Geometry: final body of the model. Coordinates: model frame, mm. A direction names the side the tool comes from. Give positions to 0.01 mm unless a question says otherwise; leave off trailing zeros. Order: outer loops, then holes, each group sorted by start corner. A loop starts at its lowest first (then second) coordinate and runs counter-clockwise, first axis right, second up. Notation, with made-up numbers: (69, 26) -> (81, 26) arc R9 ccw to (81, 36) -> close; hole circle Ø8 at (59, -36). An arc over 180 degrees is marked (long way). One line per question, with ' | ' between items.
from build123d import *

# Parameters (mm, degrees)
SKETCH_1_R          = 31.5
EXTRUDE_1_DEPTH     = 25
SKETCH_2_R          = 5
EXTRUDE_2_DEPTH     = 9
SKETCH_3_R          = 31.5
EXTRUDE_3_DEPTH     = 4
SKETCH_4_R          = 29.5
CUT_EXTRUDE_1_DEPTH = 2
SKETCH_5_R          = 8
EXTRUDE_4_DEPTH     = 30
SKETCH_6_R          = 2
CUT_EXTRUDE_2_DEPTH = 20


with BuildPart() as part:
    # 草图1 → 凸台-拉伸1 (new body)
    with BuildSketch(Plane.XY):
        Circle(SKETCH_1_R)
    extrude(amount=EXTRUDE_1_DEPTH)

    # 草图2 → 凸台-拉伸2 (add)
    with BuildSketch(Plane.XY.offset(25)):
        Circle(SKETCH_2_R)
    extrude(amount=EXTRUDE_2_DEPTH)

    # 草图3 → 凸台-拉伸3 (add)
    with BuildSketch(Plane.XY.offset(34)):
        Circle(SKETCH_3_R)
    extrude(amount=EXTRUDE_3_DEPTH)

    # 草图4 → 切除-拉伸1 (cut)
    with BuildSketch(Plane.XY.offset(38)):
        Circle(SKETCH_4_R)
    extrude(amount=-CUT_EXTRUDE_1_DEPTH, mode=Mode.SUBTRACT)

    # 草图5 → 凸台-拉伸4 (add)
    with BuildSketch(Plane.XY.offset(36)):
        Circle(SKETCH_5_R)
    extrude(amount=EXTRUDE_4_DEPTH)

    # 草图6 → 切除-拉伸2 (cut, symmetric)
    with BuildSketch(Plane(origin=(0, 0, 0), x_dir=(1, 0, 0), z_dir=(0, 1, 0))):
        with Locations(Location((0, -58, 0), (0, 0, 270))):
            Circle(SKETCH_6_R)
    extrude(amount=CUT_EXTRUDE_2_DEPTH, both=True, mode=Mode.SUBTRACT)


solid = part.part
1) Section B-B on x = 0. Return loops of the section in (y, z), plus the area to 4 significant figures.
Check result:
outline: (-31.5, 0) -> (31.5, 0) -> (31.5, 25) -> (5, 25) -> (5, 34) -> (31.5, 34) -> (31.5, 38) -> (29.5, 38) -> (29.5, 36) -> (8, 36) -> (8, 56) -> (-8, 56) -> (-8, 36) -> (-29.5, 36) -> (-29.5, 38) -> (-31.5, 38) -> (-31.5, 34) -> (-5, 34) -> (-5, 25) -> (-31.5, 25) -> close; (-8, 60) -> (8, 60) -> (8, 66) -> (-8, 66) -> close | area: 2,215 mm^2
2) Set-up query: faces 1 (the cylindrical face through (-1.08, -4.88, 29.44)), 2 (the cylindrical face through (-4.101, 31.232, 35.972)), 3 (the flat face through (6, -6, 36)). Return all of +Z, -Z, +X, -X, +Y, -Y with unobstructed straight access to the full face (end or side cutting, diameter ignored); none if empty.
Check result:
face 1: none | face 2: +Z, -Z | face 3: +Z
3) Section D-D on x = -22. Return loops of the section in (y, z), plus the area to 3 significant figures.
Check result:
outline: (-22.54, 0) -> (22.54, 0) -> (22.54, 25) -> (-22.54, 25) -> close; (-22.54, 34) -> (22.54, 34) -> (22.54, 38) -> (19.65, 38) -> (19.65, 36) -> (-19.65, 36) -> (-19.65, 38) -> (-22.54, 38) -> close | area: 1,230 mm^2
4) Section A-A on y = 0. Return loops of the section in (x, z).
Check result:
outline: (-31.5, 0) -> (31.5, 0) -> (31.5, 25) -> (5, 25) -> (5, 34) -> (31.5, 34) -> (31.5, 38) -> (29.5, 38) -> (29.5, 36) -> (8, 36) -> (8, 66) -> (-8, 66) -> (-8, 36) -> (-29.5, 36) -> (-29.5, 38) -> (-31.5, 38) -> (-31.5, 34) -> (-5, 34) -> (-5, 25) -> (-31.5, 25) -> close; hole circle Ø4 at (0, 58)
5) Section C-C on y = -18.5. Return loops of the section in (x, z), plus the area to 3 significant figures.
Check result:
outline: (-25.5, 0) -> (25.5, 0) -> (25.5, 25) -> (-25.5, 25) -> close; (-25.5, 34) -> (25.5, 34) -> (25.5, 38) -> (22.98, 38) -> (22.98, 36) -> (-22.98, 36) -> (-22.98, 38) -> (-25.5, 38) -> close | area: 1,390 mm^2
6) Contact query for flat-ended pins moving along their axis: pin 1 Ø10 at (x, y) = (-19, 22) entering from +Z; pin 2 Ø2.5 at (x, z) = (0, 58) entering from -Y; pin 3 Ø1 at (y, z) = (15, 36) entering from -X. Output: stop coordinate, or through.
Check result:
pin 1: stops at z = 38 | pin 2: passes through | pin 3: stops at x = -27.96
7) Pull-direction query (Z, two-part tool) for faces 4 (the cylindrical face through (28.14, 8.86, 37.01)), 5 (the flat face through (7, 0, 34)), 6 (the flat face through (0, 0, 66)); classes: +Z half, -Z half, draft (parallel to the pull), parting line (faces both ways), or undercut.
Check result:
face 4: draft | face 5: undercut | face 6: +Z half
8) Material intervals for probe 1 along Y at (x, z) = (0, 37); probe 2 along Z at (x, y) = (26.5, -3); probe 3 along Z at (x, y) = (0, 1), sorted ascending. Write a range as from..to.
Check result:
probe 1: y = -31.5..-29.5, -8..8, 29.5..31.5 | probe 2: z = 0..25, 34..36 | probe 3: z = 0..56, 60..66
